Here's how the part is built. I have some questions about the finished solid (model axes, mm). A direction names the side the tool comes from. Give positions to 0.01 mm unless a question says otherwise; leave off trailing zeros. Loops run counter-clockwise (first coordinate to the right, second up) from the corner with the lowest first, then second, coordinate; pieces in that order, holes last.
Q1. Suppose I cut it at A-A (y = 21). List the corners of the cut face in (x, z) for me (3 decimals).
Q2. Thinking about a two-plate mould opening in X: for faces 4 (the face through (45.8, -12.5, 38.1)), 5 (the face through (30.509, 3.913, 52.192)), 6 (the face through (-4, -7.938, 31)), 7 (the face through (20.484, 4, 18)), which applies, pulls with the +X half, pulls with the -X half, needs draft (parallel to the pull), parting line crosses it, or undercut?
Q3. Suppose I cut it at C-C (x = 80.5). List the corners of the cut face in (y, z) for me (3 decimals).
Q4. Suppose I cut it at B-B (z = 1.5). List the corners of the cut face in (x, y) for me (3 decimals), and give its area (3 significant figures).
Q5. I'm going to push flat-ended pins straight in: P1, Ø14.5, axis at x = 76, z = 57, coming from the +Y side; P2, Ø1.6, axis at x = 58, y = -8, coming from the +Z side; P3, Ø19, axis at x = 3, y = 44.5, coming from the +Z side (3 decimals). Where does each tip first touch, or does it pass through?
Q6. For faces 1 (the face through (40, 0, 37)), 2 (the face through (65, -25.4, 45)), 3 (the face through (20.484, -17, 18)), which set-ups out of +Z, -Z, +X, -X, +Y, -Y let a thin tool reach every point of the face, with its end or its side?
Q7. I need wall thicknesses on probe 1 along X at (y, z) = (-11.5, 19) (3 decimals); probe 2 along Y at (x, z) = (84, 60); probe 3 along Z at (x, y) = (17, -10) (3 decimals). Which ranges of each line are inside material? Lowest first, please.
```python
from build123d import *

# Parameters (mm, degrees)
F1_DEPTH = 63.5
F2_DEPTH = 25.4
F3_DEPTH = 7.9375
F4_DEPTH = 25.4


with BuildPart() as f1:
    # F0 (on Front) → F1 (new body, symmetric)
    with BuildSketch(Plane.XZ):
        Polygon((41.275, -9.525), (41.275, 9.525), (20.484332, 9.525), (-41.275, 9.525), (-41.275, -9.525), align=None)
    extrude(amount=F1_DEPTH, both=True)

    # F0 (on Front) → F2 (join)
    with BuildSketch(Plane.XZ):
        with BuildLine():
            Line((20.484332, 9.525), (41.275, 9.525))
            Line((41.275, 9.525), (41.275, 27.0002))
            ThreePointArc((41.275, 27.0002), (45.92468, 38.22552), (57.15, 42.8752))
            Line((57.15, 42.8752), (60.325, 42.8752))
            Line((60.325, 42.8752), (60.325, 63.665868))
            Line((60.325, 63.665868), (57.15, 63.665868))
            add(Edge.make_bspline(
                [(55.888309, 63.644154), (56.311167, 63.654873), (56.731763, 63.662127), (57.15, 63.665868)],
                knots=[111.128232, 111.128232, 111.128232, 111.128232, 112.33305, 112.33305, 112.33305, 112.33305], degree=3))
            ThreePointArc((55.888309, 63.644154), (30.781155, 52.476763), (20.484332, 27.0002))
            Line((20.484332, 27.0002), (20.484332, 9.525))
        make_face()
    extrude(amount=F2_DEPTH)

    # F0 (on Front) → F3 (join, symmetric)
    with BuildSketch(Plane.XZ):
        with BuildLine():
            Line((-41.275, 9.525), (20.484332, 9.525))
            Line((20.484332, 9.525), (20.484332, 27.0002))
            ThreePointArc((20.484332, 27.0002), (30.781155, 52.476763), (55.888309, 63.644154))
            add(Edge.make_bspline(
                [(-41.275, 9.525), (-41.352221, 32.188205), (16.885422, 62.65548), (55.888309, 63.644154)],
                knots=[0, 0, 0, 0, 111.128232, 111.128232, 111.128232, 111.128232], degree=3))
        make_face()
    extrude(amount=F3_DEPTH, both=True)

    # F0 (on Front) → F4 (join, symmetric)
    with BuildSketch(Plane.XZ):
        Polygon((60.325, 63.665868), (60.325, 42.8752), (60.325, 38.1), (111.125, 38.1), (111.125, 66.675), (60.325, 66.675), align=None)
    extrude(amount=F4_DEPTH, both=True)


solid = f1.part
```
Solutions:
1. outline: (-41.275, -9.525) - (41.275, -9.525) - (41.275, 9.525) - (-41.275, 9.525) - close; (60.325, 38.1) - (111.125, 38.1) - (111.125, 66.675) - (60.325, 66.675) - close
2. face 4: undercut
2. face 5: undercut
2. face 6: needs draft
2. face 7: pulls with the +X half
3. outline: (-25.4, 38.1) - (25.4, 38.1) - (25.4, 66.675) - (-25.4, 66.675) - close
4. outline: (-41.275, -63.5) - (41.275, -63.5) - (41.275, 63.5) - (-41.275, 63.5) - close
4. area: 10,500 mm2
5. P1: stops at y = 25.4
5. P2: stops at z = 63.67
5. P3: stops at z = 9.525
6. face 1: +Y
6. face 2: +Z, +X, -X, -Y
6. face 3: +Z, -X, -Y
7. probe 1: x = 20.484 to 41.275
7. probe 2: y = -25.4 to 25.4
7. probe 3: z = -9.525 to 9.525
